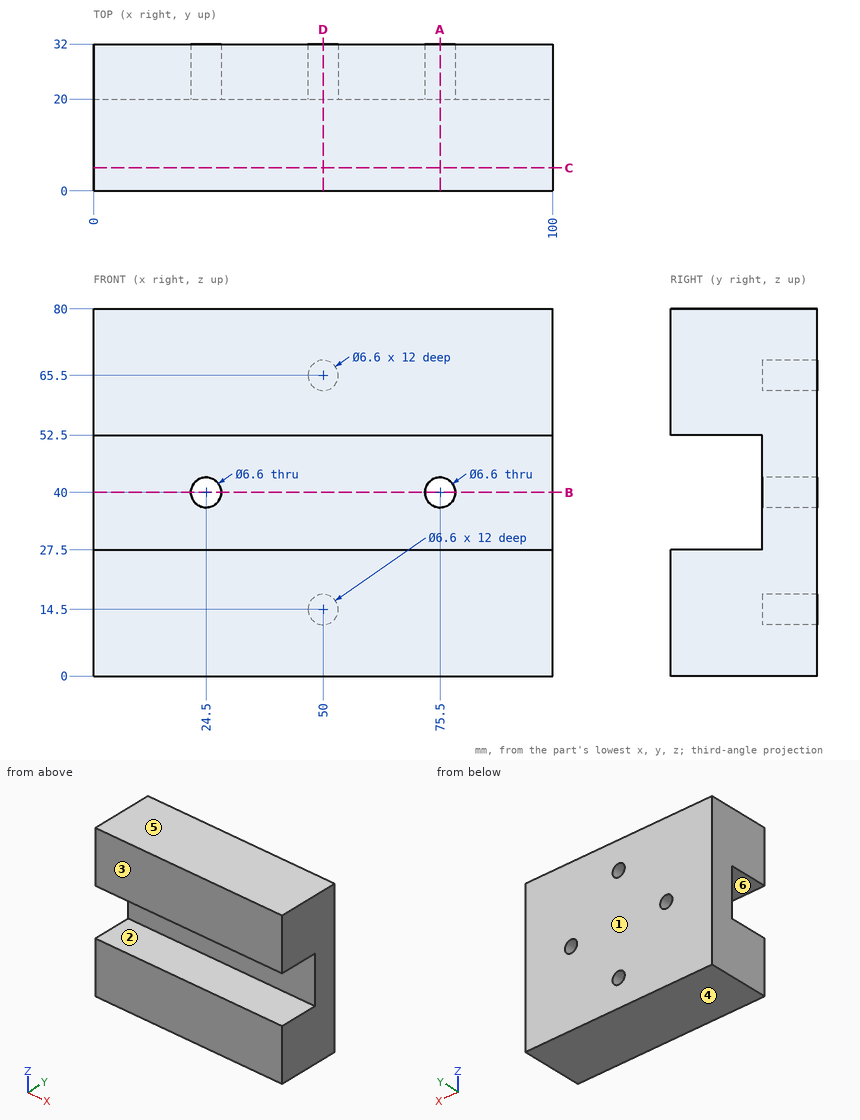
Can you work these out from the drawing? Everything is in mm from the part's minimum corner. A direction names the side the tool comes from. Give positions to 0.01 mm unless a question says otherwise; leave off trailing zeros. Order: outer loops, then holes, each group sorted by start corner. A loop starts at its lowest first (then second) coordinate and runs counter-clockwise, first axis right, second up. Notation, with made-up numbers: M 5,85.25 L 32,85.25 A8 ccw 32,94.25 Z; hole C 56,-29 d3. An arc over 180 degrees is marked long. One line per item, written item: value.
Item 1: If we section it at B-B on z = 40: Write out the boundary of the cut face in (x, y), and give its area (3 significant figures).
Verdict:
outline: M 0,20 L 21.2,20 L 21.2,32 L 0,32 Z; M 27.8,20 L 72.2,20 L 72.2,32 L 27.8,32 Z; M 78.8,20 L 100,20 L 100,32 L 78.8,32 Z
area: 1,040 mm2
Item 2: If we section it at C-C on y = 5: Write out the boundary of the cut face in (x, z), and give its area (3 significant figures).
Verdict:
outline: M 0,0 L 100,0 L 100,27.5 L 0,27.5 Z; M 0,52.5 L 100,52.5 L 100,80 L 0,80 Z
area: 5,500 mm2
Item 3: If we section it at A-A on x = 75.5: Write out the boundary of the cut face in (y, z), and give its area (3 significant figures).
Verdict:
outline: M 0,0 L 32,0 L 32,36.7 L 20,36.7 L 20,27.5 L 0,27.5 Z; M 0,52.5 L 20,52.5 L 20,43.3 L 32,43.3 L 32,80 L 0,80 Z
area: 1,980 mm2
Item 4: If we mould it in two halves opening along Z, with no side actions, what happens to the marked faces 3, 4, 5 and 6? For each: pulls with the +Z half, pulls with the -Z half, needs draft (parallel to the pull), parting line crosses it, or undercut.
Verdict:
face 3: needs draft
face 4: pulls with the -Z half
face 5: pulls with the +Z half
face 6: undercut
Item 5: For pin 1 (7.5 mm diameter, centred on x = 50, z = 16, fed in from +Y); pin 2 (3.5 mm diameter, centred on x = 51, z = 66.5, fed in from +Y); pin 3 (7.5 mm diameter, centred on x = 75.5, z = 40, fed in from -Y), each with a flat end and sliding along its axis, tell me the tip position at first contact or that it passes through.
Verdict:
pin 1: y = 32
pin 2: y = 20
pin 3: y = 20
Item 6: If we section it at D-D on x = 50: Write out the boundary of the cut face in (y, z), and give its area (3 significant figures).
Verdict:
outline: M 0,0 L 32,0 L 32,11.2 L 20,11.2 L 20,17.8 L 32,17.8 L 32,62.2 L 20,62.2 L 20,68.8 L 32,68.8 L 32,80 L 0,80 L 0,52.5 L 20,52.5 L 20,27.5 L 0,27.5 Z
area: 1,900 mm2
Item 7: Please list where these lines run through material, in increasing order: line 1 (Z direction, x = 50, y = 29); line 2 (Z direction, x = 11, y = 10); line 3 (Z direction, x = 24.5, y = 27.75).
Verdict:
line 1: 0 to 11.2, 17.8 to 62.2, 68.8 to 80
line 2: 0 to 27.5, 52.5 to 80
line 3: 0 to 36.7, 43.3 to 80
Item 8: For the marked faces 1 and 2, which set-ups out of +Z, -Z, +X, -X, +Y, -Y let a thin tool reach every point of the face, with its end or its side?
Verdict:
face 1: +Z, -Z, +X, -X, +Y
face 2: +X, -X, -Y
